Input: part model. Units: mm. Frame: model coordinates. A direction names the side the tool comes from. Give positions to 0.01 mm unless a question says otherwise; leave off trailing zeros. Loops run counter-clockwise (first coordinate to the right, second up) from the corner with the lowest first, then second, coordinate; pieces in that order, holes last. Notation, with made-up numbers: M 54,-15.5 L 82,-15.5 A15 cw 82,9.5 Z; hole C 87.5,-29 d1. An arc over 180 degrees is marked long. Answer as a JSON object with one key per item and string values. Group by question number.
1) Section query A-A on x = -19. Return loops of the section in (y, z).
2) Section query C-C on x = -27. Return loops of the section in (y, z).
3) Section query D-D on z = 61.5. Return loops of the section in (x, y).
4) Access query for faces 1 (the flat face through (-36.5, 4.9, -10)), 2 (the flat face through (-20.25, 5, 44)), 3 (the flat face through (-15.25, 5, 59)). Directions: +Z, -Z, +X, -X, +Y, -Y. A direction counts if a zero-diameter tool reaches every point of the face in a straight line with its end or side. Return the directions, or none.
5) Ray query, L1, parallel to X at y = 5, z = -6.15; L2, parallel to Z at x = 0.5, y = 2; L3, parallel to Y at x = 16.5, z = 61.5. Return the intervals inside material, ascending.
6) Section query B-B on z = -6. Return loops of the section in (x, y).
7) Draft query along X for faces 4 (the flat face through (15.25, 5, 59)), 5 (the flat face through (29, 5, 0)), 6 (the flat face through (-27, 5, 16.5)), 7 (the flat face through (-39, 5, -8)). Return one class per face: +X half, -X half, draft (parallel to the pull), parting line (faces both ways), or undercut.
8) First-contact query: P1, Ø3, axis at x = 7.5, y = 6.5, coming from the +Z side; P2, Ø1, axis at y = 8.5, z = 45.5, coming from the +X side; P3, Ø4, axis at x = -36, y = 6.5, coming from the -Z side; P4, Ø3, axis at x = -2, z = 34.5, coming from the -Y side. Flat tips, straight axial feed; report the tip coordinate or a pass-through.
from build123d import *

# Parameters (mm, degrees)
CROQUIS1_W                 = 58
CROQUIS1_H                 = 33
CROQUIS1_W_2               = 50
CROQUIS1_H_2               = 25
SALIENTE_EXTRUIR1_DEPTH    = 10
REDONDEO1_R                = 5
REDONDEO2_R                = 5
CROQUIS2_R                 = 2.3
CORTAR_EXTRUIR1_DEPTH      = 52
CROQUIS3_W                 = 4
CROQUIS3_H                 = 10
CORTAR_EXTRUIR2_DEPTH      = 20
CROQUIS4_W                 = 5
CROQUIS4_H                 = 10
SALIENTE_EXTRUIR2_DEPTH    = 10
REDONDEO3_R                = 5
REDONDEO4_R                = 5
CORTAR_EXTRUIR4_DEPTH      = 27
CORTAR_EXTRUIR4_DEPTH_BACK = 27
CROQUIS5_R                 = 2.2


with BuildPart() as part:
    # Croquis1 → Saliente-Extruir1 (new body)
    # profile 1 of 2: a face of its own
    with BuildSketch(Plane(origin=(0, 0, 0), x_dir=(1, 0, 0), z_dir=(0, 1, 0))):
        Rectangle(CROQUIS1_W, CROQUIS1_H)
        Rectangle(CROQUIS1_W_2, CROQUIS1_H_2, mode=Mode.SUBTRACT)
    # profile 2 of 2: a face of its own
    with BuildSketch(Plane(origin=(0, 0, 0), x_dir=(1, 0, 0), z_dir=(0, 1, 0))):
        Polygon((20.25, -16.5), (-20.25, -16.5), (-20.25, -66.5), (-15.25, -66.5), (-15.25, -51.5), (15.25, -51.5), (15.25, -66.5), (20.25, -66.5), align=None)
    extrude(amount=SALIENTE_EXTRUIR1_DEPTH)

    # Redondeo1
    redondeo1_edges = [part.edges().sort_by_distance(p)[0] for p in [
        (20.25, 5, 16.5),
    ]]
    fillet(redondeo1_edges, radius=REDONDEO1_R)

    # Redondeo2
    redondeo2_edges = [part.edges().sort_by_distance(p)[0] for p in [
        (-20.25, 5, 16.5),
    ]]
    fillet(redondeo2_edges, radius=REDONDEO2_R)

    # Croquis2 → Cortar-Extruir1 (cut)
    with BuildSketch(Plane.ZY.offset(20.25)):
        with Locations((61.5, 5)):
            Circle(CROQUIS2_R)
    extrude(amount=-CORTAR_EXTRUIR1_DEPTH, mode=Mode.SUBTRACT)

    # Croquis3 → Cortar-Extruir2 (cut)
    with BuildSketch(Plane.XZ):
        with Locations((-27, 0)):
            Rectangle(CROQUIS3_W, CROQUIS3_H)
    extrude(amount=-CORTAR_EXTRUIR2_DEPTH, mode=Mode.SUBTRACT)

    # Croquis4 → Saliente-Extruir2 (add)
    with BuildSketch(Plane.ZY.offset(29)):
        with Locations((-7.5, 5)):
            Rectangle(CROQUIS4_W, CROQUIS4_H)
        with Locations((7.5, 5)):
            Rectangle(CROQUIS4_W, CROQUIS4_H)
    extrude(amount=SALIENTE_EXTRUIR2_DEPTH)

    # Redondeo3
    redondeo3_edges = [part.edges().sort_by_distance(p)[0] for p in [
        (-29, 5, -10),
    ]]
    fillet(redondeo3_edges, radius=REDONDEO3_R)

    # Redondeo4
    redondeo4_edges = [part.edges().sort_by_distance(p)[0] for p in [
        (-29, 5, 10),
    ]]
    fillet(redondeo4_edges, radius=REDONDEO4_R)

    # Croquis5 → Cortar-Extruir4 (cut, two sides: drawn at the far end of the back side and taken through both)
    with BuildSketch(Plane.XY.offset(10).offset(-CORTAR_EXTRUIR4_DEPTH_BACK)):
        with Locations(Location((-34, 5, 0), (0, 0, 90))):
            Circle(CROQUIS5_R)
    extrude(amount=CORTAR_EXTRUIR4_DEPTH + CORTAR_EXTRUIR4_DEPTH_BACK, mode=Mode.SUBTRACT)


solid = part.part
Output:
{
 "1": {"outline": "M 0,-16.5 L 10,-16.5 L 10,-12.5 L 0,-12.5 Z; M 0,12.5 L 10,12.5 L 10,66.5 L 0,66.5 Z; hole C 5,61.5 d4.6"},
 "2": {"outline": "M 0,-16.5 L 10,-16.5 L 10,-5 L 0,-5 Z; M 0,5 L 10,5 L 10,16.5 L 0,16.5 Z"},
 "3": {"outline": "M -20.25,0 L -15.25,0 L -15.25,2.7 L -20.25,2.7 Z; M -20.25,7.3 L -15.25,7.3 L -15.25,10 L -20.25,10 Z; M 15.25,0 L 20.25,0 L 20.25,2.7 L 15.25,2.7 Z; M 15.25,7.3 L 20.25,7.3 L 20.25,10 L 15.25,10 Z"},
 "4": {"face 1": "-Z, -X, +Y, -Y", "face 2": "+Z, -X, +Y, -Y", "face 3": "+Z, +Y, -Y"},
 "5": {"L1": "x = -39 to -36.2, -31.8 to -25, 25 to 29", "L2": "z = -16.5 to -12.5, 12.5 to 51.5", "L3": "y = 0 to 2.7, 7.3 to 10"},
 "6": {"outline": "M -39,0 L -25,0 L -25,10 L -39,10 Z; M 25,0 L 29,0 L 29,10 L 25,10 Z; hole C -34,5 d4.4"},
 "7": {"face 4": "undercut", "face 5": "+X half", "face 6": "draft", "face 7": "-X half"},
 "8": {"P1": "stops at z = 51.5", "P2": "stops at x = 20.25", "P3": "stops at z = -10", "P4": "stops at y = 0"}
}
